Source: three-view drawing plus pictorial views. Frame: mm from the lowest corner of the part. A direction names the side the tool comes from. Give positions to 0.01 mm unless a question says otherwise; leave off trailing zeros. Loops run counter-clockwise (first coordinate to the right, second up) from the corner with the lowest first, then second, coordinate; pieces in that order, holes last. Notation, with made-up numbers: (-40, 44.25) - (-15, 44.25) arc R37 cw to (-15, 81.25) - close; hole circle Ø10 at (4, 79). An arc over 180 degrees is marked (long way). Answer in a Markdown table with one row per item.
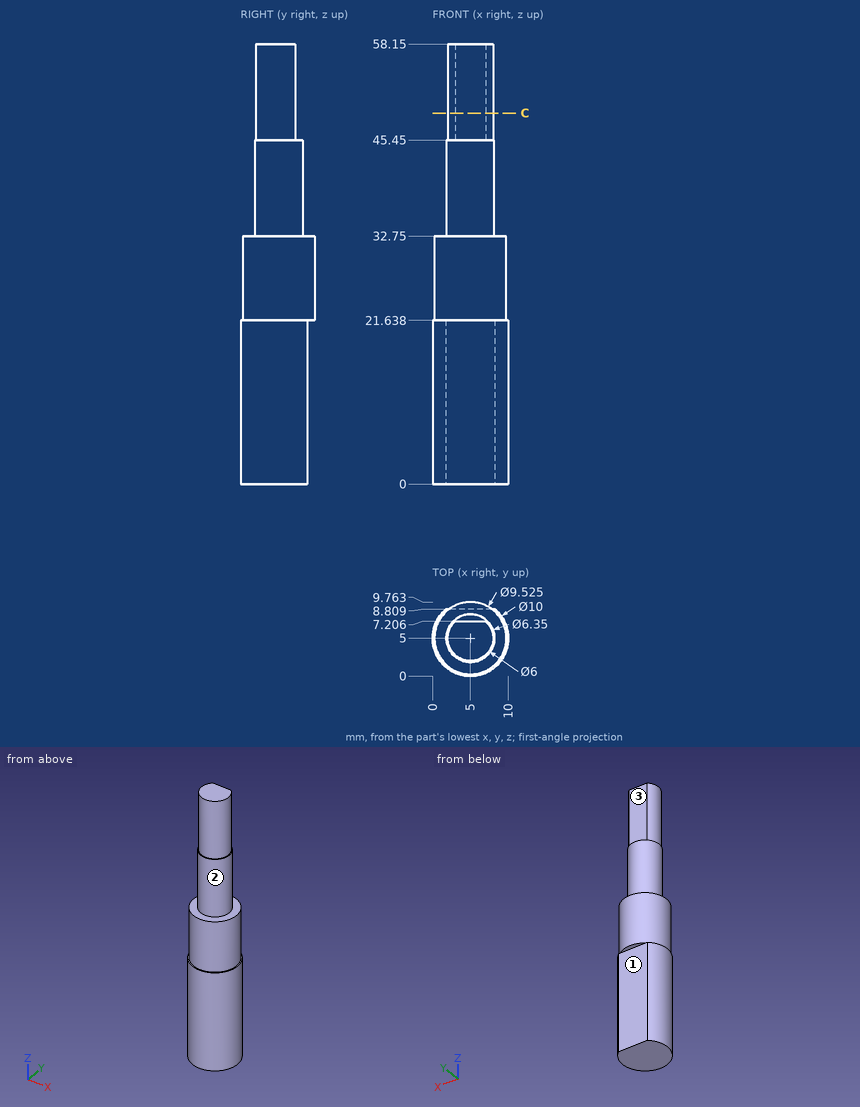
Q1. Material intervals for line 1 along Z through (x, y) = (5.75, 0.5); line 2 along Z through (x, y) = (4.5, 9.25); line 3 along Y through (x, z) = (4.75, 48), sorted ascending.
Check values:
| item | result |
|---|---|
| line 1 | 0 to 32.75 |
| line 2 | 21.64 to 32.75 |
| line 3 | 2.01 to 7.21 |
Q2. Reachability of the marked faces 1, 2 and 3 from +Z, -Z, +X, -X, +Y, -Y: full face, straight path, thin tool, end or side. Return the list, or none.
Check values:
| item | result |
|---|---|
| face 1 | -Z, +X, -X, +Y |
| face 2 | +Z |
| face 3 | +Z, +X, -X, +Y |
Q3. Cut plane C-C (z = 49). Output: boundary loops of the cut face in (x, y).
Check values:
| item | result |
|---|---|
| outline | (2.97, 7.21) arc R3 ccw (long way) to (7.03, 7.21) - close |
Q4. First-contact query: pin 1 (3 mm diameter, centred on x = 3.5, z = 8.5, fed in from +Y); pin 2 (1 mm diameter, centred on x = 5.5, y = 9.5, fed in from -Z); pin 3 (5 mm diameter, centred on y = 1.5, z = 43, fed in from +X). Flat tips, straight axial feed; report the tip coordinate or a pass-through.
Check values:
| item | result |
|---|---|
| pin 1 | y = 8.81 |
| pin 2 | z = 21.64 |
| pin 3 | x = 8.01 |
